Autodesk Inventor part; units mm, degrees
ref_plane "YZ Plane" through (0, 0, 0) normal (1, 0, 0) x (0, 1, 0)
ref_plane "XZ Plane" through (0, 0, 0) normal (0, 1, 0) x (-1, 0, 0)
ref_plane "XY Plane" through (0, 0, 0) normal (0, 0, 1) x (1, 0, 0)
sketch "Sketch1" plane through (0, 0, 0) normal (1, 0, 0) x (0, 1, 0)
  line L0 (0, 0) -> (0, -15.044)
  line L1 (2.5, 0) -> (2.5, -12.9861)
  line L2 (0, -7.522) -> (12, -7.522) construction
  line L3 (0, -1.512) -> (12, -1.512) construction
  line L4 (12, -1.512) -> (9.805, 0.683)
  line L5 (12, -7.522) -> (9.805, -9.717)
  line L6 (12, -1.512) -> (9.805, -3.707)
  line L7 (12, -7.522) -> (9.805, -5.327)
  line L8 (9.805, -5.327) -> (9.805, -3.707)
  line L9 (9.805, 0.683) -> (2.5, 0.683)
  line L10 (2.5, 0.683) -> (2.5, 0)
  line L11 (9.805, -9.717) -> (2.5, -9.717)
  dimension "d0" = 2.5
  dimension "d1" = 12
  dimension "d2" = 6.01
  dimension "d3" = 45
  dimension "d4" = 0
  dimension "d5" = 10.4
revolve "Revolution1" add sketch "Sketch1" angle 360 about axis through (0, 0, 0) along (0, 0, -1)
properties part number "bearingType2Standin"
Can you work these out from the model? Positions are in its coordinate system, mm. A direction names the side the tool comes from. Round coordinates to 2 decimals unless told otherwise and drop trailing zeros. Write each loop counter-clockwise with the first axis right and the second up, starting at its lowest first coordinate (ties: lowest second). Pieces come first, ordered by that corner, then holes. Notation, with made-up numbers: (-37.5, 88) -> (-5.5, 88) arc R25 ccw to (-5.5, 106) -> close; hole circle Ø5 at (49.5, 16). An arc over 180 degrees is marked (long way). Use one line per item in the form item = value. Start each with the question number.
Q1. We'd pull the mould along Y, two halves only. Please class faces 3 (the face through (-2.44, -0.54, -4.59)), 4 (the face through (-2, 2, -9.717)), 5 (the face through (-2.95, 9.35, -4.51)): +Y half, -Y half, draft (parallel to the pull), parting line (faces both ways), or undercut.
Q2. Imagine slicing it at C-C (z = -4.75). Please give me the cut outline in (x, y) (3 decimals), then the cut area to 3 significant figures.
Q3. Imagine slicing it at A-A (y = 0). Please give me the cut outline in (x, z) (3 decimals), then the cut area to 3 significant figures.
Q4. If I drill on probe 1 along X at (y, z) = (0, -5) (3 decimals); probe 2 along Z at (x, y) = (6.5, 8); probe 3 along Y at (x, z) = (1.75, -6.5), over which ranges is the centre line in solid material (lowest first)? Write a range as [from, to].
Q5. Imagine slicing it at D-D (z = 0). Please give me the cut outline in (x, y).
Q6. Which directions (+Z, -Z, +X, -X, +Y, -Y) give clear straight access to the entire face, cutting with the end or side of a thin tool? Please do faces 1 (the face through (-9.706, -2.155, -5.464)), 2 (the face through (-9.706, -2.155, 0.546)).
Q7. I'm going to push flat-ended pins straight in: P1, Ø1, axis at y = 4, z = -4, coming from the +X side; P2, Ø3, axis at x = 0, y = 0, coming from the -Z side; P3, Ø1.5, axis at x = -8, z = -1, coming from the +Y side. Where does each tip first touch, or does it pass through?
Worked out:
q1.face_3 = undercut
q1.face_4 = draft
q1.face_5 = parting line
q2.outline = circle Ø19.61 at (0, 0); hole circle Ø5 at (0, 0)
q2.area = 282 mm^2
q3.outline = (-12, -7.522) -> (-9.805, -9.717) -> (-2.5, -9.717) -> (-2.5, 0.683) -> (-9.805, 0.683) -> (-12, -1.512) -> (-9.805, -3.707) -> (-9.805, -5.327) -> close; (2.5, -9.717) -> (9.805, -9.717) -> (12, -7.522) -> (9.805, -5.327) -> (9.805, -3.707) -> (12, -1.512) -> (9.805, 0.683) -> (2.5, 0.683) -> close
q3.area = 171 mm^2
q4.probe_1 = [-9.805, -2.5], [2.5, 9.805]
q4.probe_2 = [-9.21, -5.83], [-3.2, 0.18]
q4.probe_3 = [-10.84, -1.79], [1.79, 10.84]
q5.outline = circle Ø20.98 at (0, 0); hole circle Ø5 at (0, 0)
q6.face_1 = none
q6.face_2 = +Z
q7.P1 = 9.22
q7.P2 = through
q7.P3 = 9.41
